Can you work these out from the model? Positions are in its coordinate system, mm. Coordinates: 2 decimals unless noted, no trailing zeros. Order: outer loops, then holes, each group sorted by start corner. A loop starts at its lowest first (then second) coordinate and runs counter-clockwise, first axis right, second up. Notation, with made-up numbers: (-38, 30.5) -> (-9, 30.5) arc R27 cw to (-9, 48.5) -> close; hole circle Ø6 at (85, 53). An arc over 180 degrees is marked (long way). Answer in a Markdown table with one row per item. Add a question column.
1. Will these pins go through, and if not, where does the flat tip stop? pin 1 (1.5 mm diameter, centred on x = -0.5, y = -2, fed in from -Z); pin 2 (1.5 mm diameter, centred on y = 9, z = 2.5, fed in from +X); pin 3 (1.5 mm diameter, centred on y = 22.5, z = 0.5, fed in from -X); pin 4 (4.5 mm diameter, centred on x = 25.4, y = 0, fed in from -Z).
2. Imagine slicing it at D-D on z = 1.5. Write out the boundary of the cut face in (x, y) (3 decimals).
3. If I drill on line 1 along X through (y, z) = (-1, 2.9); line 2 along Y through (x, z) = (6.5, 1.05); line 3 along X through (y, z) = (25, 0.45), over which ranges is the centre line in solid material (lowest first)? Write a range as [from, to].
4. We'd pull the mould along Y, two halves only. Please class faces 1 (the face through (-1.915, 1.468, 1.565)), 2 (the face through (13, 5, 3.175)), 3 (the face through (14, -12.7, 2)): pulls with the +Y half, pulls with the -Y half, needs draft (parallel to the pull), parting line crosses it, or undercut.
5. Imagine slicing it at A-A on y = 0. Write out the boundary of the cut face in (x, z) (3 decimals), plus the area to 3 significant figures.
6. Imagine slicing it at C-C on y = 25.4. Write out the boundary of the cut face in (x, z) (3 decimals).
7. Imagine slicing it at B-B on x = 8. Write out the boundary of the cut face in (y, z) (3 decimals).
Autodesk Inventor part; units mm, degrees
ref_plane "YZ Plane" through (0, 0, 0) normal (1, 0, 0) x (0, 1, 0)
ref_plane "XZ Plane" through (0, 0, 0) normal (0, 1, 0) x (-1, 0, 0)
ref_plane "XY Plane" through (0, 0, 0) normal (0, 0, 1) x (1, 0, 0)
sketch "Sketch1" plane through (0, 0, 0) normal (0, 0, 1) x (1, 0, 0)
  circle A0 centre (0, 0) radius 2.413
  circle A1 centre (25.4, 0) radius 2.413
  line L0 (25.4, 0) -> (0, 0) construction
  line L1 (-5.08, 6.35) -> (31.75, 6.35) construction
  line L2 (31.75, 6.35) -> (31.75, -12.7)
  line L3 (31.75, -12.7) -> (-5.08, -12.7)
  line L4 (-5.08, -12.7) -> (-5.08, 6.35)
  line L5 (-5.08, 6.35) -> (1.5668, 27.3188)
  line L6 (31.75, 6.35) -> (12.4993, 29.4638)
  circle A2 centre (7.62, 25.4) radius 2.4638
  arc A3 (12.4993, 29.4638) -> (1.5668, 27.3188) centre (7.62, 25.4) ccw
  line L7 (-5.08, -12.7) -> (-5.08, 6.35)
  line L8 (-5.08, -12.7) -> (31.75, -12.7)
  line L9 (31.75, -12.7) -> (31.75, 6.35)
  line L10 (31.75, 6.35) -> (12.4993, 29.4638)
  dimension "d1" = 4.826
  dimension "d5" = 12.7
  dimension "d6" = 6.35
  dimension "d7" = 5.08
  dimension "d9" = 6.35
  dimension "d10" = 25.4
  dimension "d14" = 12.7
  dimension "d15" = 19.05
  dimension "d16" = 4.9276
  dimension "d17" = 6.35
extrude "Extrusion1" add sketch "Sketch1" along normal blind 3.175
fillet "Fillet1" radius 3.175 2 edges at (31.75, 6.35, 1.5875) (-5.08, 6.35, 1.5875)
properties part number "Bracket" material "Aluminum 6061"
Answers follow:
| question | item | result |
|---|---|---|
| 1 | pin 1 | stops at z = 0 |
| 1 | pin 2 | stops at x = 30.17 |
| 1 | pin 3 | stops at x = -0.2 |
| 1 | pin 4 | passes through |
| 2 | outline | (-5.08, -12.7) -> (31.75, -12.7) -> (31.75, 5.201) arc R3.175 ccw to (31.015, 7.233) -> (12.499, 29.464) arc R6.35 ccw to (1.567, 27.319) -> (-4.932, 6.818) arc R3.175 ccw to (-5.08, 5.859) -> close; hole circle Ø4.826 at (0, 0); hole circle Ø4.928 at (7.62, 25.4); hole circle Ø4.826 at (25.4, 0) |
| 3 | line 1 | x = [-5.08, -2.2], [2.2, 23.2], [27.6, 31.75] |
| 3 | line 2 | y = [-12.7, 23.21], [27.59, 31.65] |
| 3 | line 3 | x = [0.83, 5.19], [10.05, 16.22] |
| 4 | face 1 | undercut |
| 4 | face 2 | needs draft |
| 4 | face 3 | pulls with the -Y half |
| 5 | outline | (-5.08, 0) -> (-2.413, 0) -> (-2.413, 3.175) -> (-5.08, 3.175) -> close; (2.413, 0) -> (22.987, 0) -> (22.987, 3.175) -> (2.413, 3.175) -> close; (27.813, 0) -> (31.75, 0) -> (31.75, 3.175) -> (27.813, 3.175) -> close |
| 5 | area | 86.3 mm² |
| 6 | outline | (0.959, 0) -> (5.156, 0) -> (5.156, 3.175) -> (0.959, 3.175) -> close; (10.084, 0) -> (15.884, 0) -> (15.884, 3.175) -> (10.084, 3.175) -> close |
| 7 | outline | (-12.7, 0) -> (22.966, 0) -> (22.966, 3.175) -> (-12.7, 3.175) -> close; (27.834, 0) -> (31.739, 0) -> (31.739, 3.175) -> (27.834, 3.175) -> close |
